Could you check a few things on this model? Use its own coordinates, in mm. A direction names the side the tool comes from. Coordinates: 2 decimals unless noted, no trailing zeros. Write each loop counter-clockwise with the first axis right and the second up, starting at its lowest first coordinate (ties: lowest second). Pieces come first, ordered by that corner, then holes. Notation, with made-up numbers: (35.5, 10.5) - (75.5, 10.5) arc R22 ccw to (75.5, 35.5) - close; hole circle Ø7 at (16.5, -29.5). An arc over 180 degrees is marked (long way). Answer as a JSON object with one key per item and string values. Group by question number.
1) We'd pull the mould along X, two halves only. Please class faces 6 (the flat face through (0, 11, -2)), 7 (the flat face through (2.413, 11, -2)), 8 (the flat face through (56, 11, -3.81)): released by +X, released by -X, zero draft, split by the parting line, or undercut.
2) If we section it at C-C (y = 14.5): Write out the boundary of the cut face in (x, z).
3) Will these pins go through, and if not, where does the flat tip stop? pin 1 Ø10 at (y, z) = (9.5, -9) entering from -X; pin 2 Ø12 at (y, z) = (3, -19) entering from +X; pin 3 Ø5 at (x, y) = (35.5, 12) entering from +Z.
4) If we section it at A-A (z = -15): Write out the boundary of the cut face in (x, y).
5) On a 3-axis mill with a long thin cutter (end or side, diameter ignored), from which of +Z, -Z, +X, -X, +Y, -Y can I reach the whole of each face in a straight line? I mean faces 1 (the flat face through (33, 0, -21)), 2 (the flat face through (50.8, 11, -10)), 3 (the flat face through (9, 11, -3.81)), 4 (the flat face through (32, 11, -23.876)), 5 (the flat face through (57.023, 11, -2)). Say none if no direction works.
6) If we section it at B-B (x = 5.08): Write out the boundary of the cut face in (y, z).
7) If we section it at D-D (y = 18.25): Write out the boundary of the cut face in (x, z), plus the area to 3 significant figures.
8) Please list where these lines run through material, in increasing order: line 1 along X through (y, z) = (3.75, -10.5); line 2 along Z through (x, y) = (25.5, 9.25); line 3 along Z through (x, y) = (8.5, 15).
```python
from build123d import *

# Parameters (mm, degrees)
BASE_DEPTH     = 21.59
BOLTHOLE_REACH = 45.79


with BuildPart() as part:
    # Sketch4 → base (new body)
    with BuildSketch(Plane(origin=(0, 0, 0), x_dir=(1, 0, 0), z_dir=(0, 1, 0))):
        Polygon((0, 0), (13.97, 0), (13.97, 20.066), (32.385, 20.066), (32.385, 23.876), (10.16, 23.876), (10.16, 3.81), (0, 3.81), align=None)
    base = extrude(amount=BASE_DEPTH)

    # Sketch5 → bolthole (cut, up to next)
    with BuildSketch(Plane(origin=(0, 0, -3.81), x_dir=(-1, 0, 0), z_dir=(0, 0, -1)), mode=Mode.PRIVATE) as bolthole_sk1:
        with BuildLine():
            Line((-2.413, 13.335), (-2.413, 8.255))
            ThreePointArc((-2.413, 8.255), (-5.08, 5.588), (-7.747, 8.255))
            Line((-7.747, 8.255), (-7.747, 13.335))
            ThreePointArc((-7.747, 13.335), (-5.08, 16.002), (-2.413, 13.335))
        make_face()
    bolthole_tool1 = extrude(bolthole_sk1.sketch, amount=-BOLTHOLE_REACH, mode=Mode.PRIVATE) & part.part
    bolthole = bolthole_tool1.solids().sort_by_distance((5.08, 10.795, -3.81))[0]
    add(bolthole, mode=Mode.SUBTRACT)

    # Mirror1: base, bolthole across plane
    add(base.mirror(Plane(origin=(32.385, 21.59, -20.066), x_dir=(0, 0, 1), z_dir=(-1, 0, 0))))
    add(bolthole.mirror(Plane(origin=(32.385, 21.59, -20.066), x_dir=(0, 0, 1), z_dir=(-1, 0, 0))), mode=Mode.SUBTRACT)


solid = part.part
```
Here are the results:
{
 "1": {"face 6": "released by -X", "face 7": "undercut", "face 8": "zero draft"},
 "2": {"outline": "(0, -3.81) - (2.68, -3.81) - (2.68, 0) - (0, 0) - close; (7.48, -3.81) - (10.16, -3.81) - (10.16, -23.88) - (54.61, -23.88) - (54.61, -3.81) - (57.29, -3.81) - (57.29, 0) - (50.8, 0) - (50.8, -20.07) - (13.97, -20.07) - (13.97, 0) - (7.48, 0) - close; (62.09, -3.81) - (64.77, -3.81) - (64.77, 0) - (62.09, 0) - close"},
 "3": {"pin 1": "stops at x = 10.16", "pin 2": "stops at x = 54.61", "pin 3": "stops at z = -20.07"},
 "4": {"outline": "(10.16, 0) - (13.97, 0) - (13.97, 21.59) - (10.16, 21.59) - close; (50.8, 0) - (54.61, 0) - (54.61, 21.59) - (50.8, 21.59) - close"},
 "5": {"face 1": "+Z, -Z, +X, -X, -Y", "face 2": "+Z, +Y, -Y", "face 3": "-Z, -X, +Y, -Y", "face 4": "-Z, +X, -X, +Y, -Y", "face 5": "+Z, -Z"},
 "6": {"outline": "(0, -3.81) - (5.59, -3.81) - (5.59, 0) - (0, 0) - close; (16, -3.81) - (21.59, -3.81) - (21.59, 0) - (16, 0) - close"},
 "7": {"outline": "(0, -3.81) - (10.16, -3.81) - (10.16, -23.88) - (54.61, -23.88) - (54.61, -3.81) - (64.77, -3.81) - (64.77, 0) - (50.8, 0) - (50.8, -20.07) - (13.97, -20.07) - (13.97, 0) - (0, 0) - close", "area": "400 mm²"},
 "8": {"line 1": "x = 10.16 to 13.97, 50.8 to 54.61", "line 2": "z = -23.88 to -20.07", "line 3": "z = -3.81 to 0"}
}
